Geometry: final body of the model. Coordinates: model frame, mm. Give positions to 0.01 mm unless a question says otherwise; leave off trailing zeros. Write each loop counter-clockwise with the first axis right and the second up, starting at its lowest first coordinate (ties: lowest second). Pieces come first, ordered by that corner, then holes. Notation, with made-up numbers: (40.5, 50.5) -> (68.5, 50.5) arc R22 ccw to (68.5, 69.5) -> close; hole circle Ø7 at (2, 82.5). An arc over 180 degrees is marked (long way). Use CSV: the item, a comma, the result in double quotes. Start each with the question number.
1) Contact query for flat-ended pins moving along their axis: P1, Ø1.5, axis at x = 53.5, y = -4.5, coming from the -Z side; P2, Ø12, axis at x = 93.5, z = 750.5, coming from the +Y side; P3, Ø5.5, axis at x = 2, y = -4, coming from the -Z side. Output: stop coordinate, or through.
2) Section A-A (z = 765). Output: boundary loops of the cut face in (x, y).
3) Material intervals for line 1 (X direction, y = 13.75, z = 765); line 2 (Z direction, x = 146, y = -1); line 3 (Z direction, x = 5, y = -13), sorted ascending. Write a range as [from, to].
4) Section D-D (y = 12). Output: boundary loops of the cut face in (x, z), plus the area to 3 significant figures.
5) Section B-B (y = 0). Output: boundary loops of the cut face in (x, z).
6) Section C-C (x = 5). Output: boundary loops of the cut face in (y, z).
```python
from build123d import *

# Parameters (mm, degrees)
CYLINDER137_R          = 3
CYLINDER137_DEPTH      = 60
CYLINDER137_ROLL_ANGLE = 90
BOX079_W               = 40
BOX079_H               = 18
BOX079_DEPTH           = 18
CYLINDER_R             = 20
CYLINDER_DEPTH         = 200
CYLINDER_PITCH_ANGLE   = 90


with BuildPart() as cilindro091:
    # Cylinder137 → Cylinder137 (new body)
    with BuildSketch(Plane.XY):
        Circle(CYLINDER137_R)
    extrude(amount=CYLINDER137_DEPTH)


with BuildPart() as cilindro091_1:
    # Cylinder137 roll: moved
    add(cilindro091.part.rotate(Axis((0, 0, 0), (1, 0, 0)), CYLINDER137_ROLL_ANGLE))


with BuildPart() as cilindro091_2:
    # Cylinder137 placement: moved
    add(cilindro091_1.part.moved(Location((5, 37, 765))))


with BuildPart() as cubo056:
    # Box079 → Box079 (new body)
    with BuildSketch(Plane(origin=(-10, -9, 755), x_dir=(1, 0, 0), z_dir=(0, 0, 1))):
        with Locations((20, 9)):
            Rectangle(BOX079_W, BOX079_H)
    extrude(amount=BOX079_DEPTH)


with BuildPart() as cut144:
    # Cylinder → Cylinder (new body)
    with BuildSketch(Plane.XY):
        Circle(CYLINDER_R)
    extrude(amount=CYLINDER_DEPTH)


with BuildPart() as cut144_1:
    # Cylinder pitch: moved
    add(cut144.part.rotate(Axis((0, 0, 0), (0, 1, 0)), CYLINDER_PITCH_ANGLE))


with BuildPart() as cut144_2:
    # Cylinder placement: moved
    add(cut144_1.part.moved(Location((-10, 0, 765))))

    # Cut143: cut Cubo056
    add(cubo056.part, mode=Mode.SUBTRACT)

    # Cut144: cut Cilindro091
    add(cilindro091_2.part, mode=Mode.SUBTRACT)


solid = cut144_2.part
```
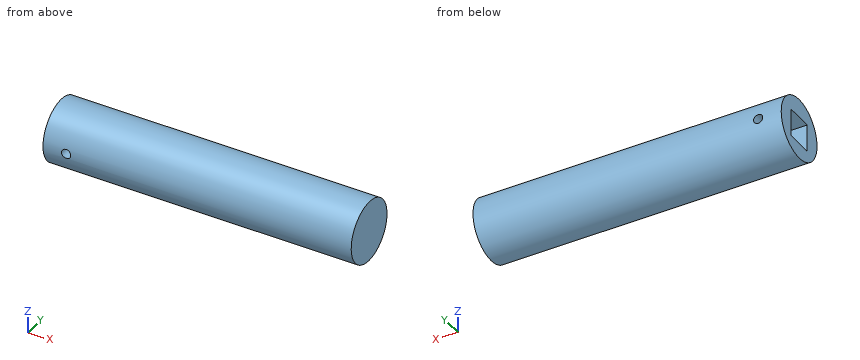
Answers follow:
1,P1,"stops at z = 745.35"
1,P2,"stops at y = 18.1"
1,P3,"stops at z = 745.04"
2,outline,"(-10, -20) -> (2, -20) -> (2, -9) -> (-10, -9) -> close; (-10, 9) -> (2, 9) -> (2, 20) -> (-10, 20) -> close; (8, -20) -> (190, -20) -> (190, 20) -> (8, 20) -> (8, 9) -> (30, 9) -> (30, -9) -> (8, -9) -> close"
3,line 1,"x = [-10, 2], [8, 190]"
3,line 2,"z = [745.03, 784.97]"
3,line 3,"z = [749.8, 762], [768, 780.2]"
4,outline,"(-10, 749) -> (190, 749) -> (190, 781) -> (-10, 781) -> close; hole circle Ø6 at (5, 765)"
4,area,"6,370 mm^2"
5,outline,"(-10, 745) -> (190, 745) -> (190, 785) -> (-10, 785) -> (-10, 773) -> (30, 773) -> (30, 755) -> (-10, 755) -> close"
6,outline,"(-19.77, 762) arc R20 ccw to (19.77, 762) -> (9, 762) -> (9, 755) -> (-9, 755) -> (-9, 762) -> close; (-19.77, 768) -> (-9, 768) -> (-9, 773) -> (9, 773) -> (9, 768) -> (19.77, 768) arc R20 ccw to start"
